Read the model definition and answer for the solid it produces. Units are mm, in the model's axes. Coordinates: 2 decimals unless noted, no trailing zeros. Order: outer loops, then holes, each group sorted by start corner. A loop starts at its lowest first (then second) coordinate and runs counter-clockwise, first axis right, second up. Notation, with made-up numbers: M 7,60.5 L 20,60.5 A13 cw 20,66.5 Z; hole C 2.5,-37 d5. An arc over 180 degrees is marked long. One line per question, with ' | ' between items. Start each with the question number.
1) Find section B-B, the plane z = -65. Write down the section's boundary in (x, y).
2) Find section A-A, the plane z = 0. Write down the section's boundary in (x, y).
3) Find section C-C, the plane z = -35.5. Write down the section's boundary in (x, y), plus the area to 3 significant figures.
4) Consider probe 1 along Z at (x, y) = (84.5, 0.3) (3 decimals); probe 2 along X at (y, z) = (0.75, 0); probe 3 along Z at (x, y) = (70.5, 0.45) (3 decimals). Determine where each line is inside the solid, lowest interval first.
from build123d import *

# Parameters (mm, degrees)
SKETCH6_R          = 1.6
EXTRUDE1_DEPTH     = 0.9
FILLET1_R          = 2
SKETCH9_R          = 0.925
CUT_EXTRUDE1_DEPTH = 1.9
CUT_EXTRUDE2_DEPTH = 1.9


with BuildPart() as part:
    # Sketch6 → Extrude1 (new body)
    with BuildSketch(Plane(origin=(0, 0, 0), x_dir=(1, 0, 0), z_dir=(0, 1, 0))):
        Polygon((-4.8675, 77.0686), (-4.8675, 62.335), (1.8535, 62.335), (1.8535, 12.335), (-4.8675, 12.335), (-4.8675, -10.395), (31.1875, -10.395), (31.1875, -7.244), (54.5375, -7.244), (54.5375, -10.395), (90.5925, -10.395), (90.5925, 25.66), (87.4415, 25.66), (87.4415, 49.01), (90.5925, 49.01), (90.5925, 83.6934), (78.5925, 83.6934), (78.5925, 80.9186), (19.1449, 80.9186), (19.1449, 75.196571572), (9.1325, 75.196571572), (5.1325, 77.0686), align=None)
        with Locations((0, 73.66)):
            Circle(SKETCH6_R, mode=Mode.SUBTRACT)
        with Locations((85.725, 76.2)):
            Circle(SKETCH6_R, mode=Mode.SUBTRACT)
        Circle(SKETCH6_R, mode=Mode.SUBTRACT)
        with Locations((85.725, -3.81)):
            Circle(SKETCH6_R, mode=Mode.SUBTRACT)
    extrude(amount=EXTRUDE1_DEPTH)

    # Fillet1
    fillet1_edges = [part.edges().sort_by_distance(p)[0] for p in [
        (5.1325, 0.45, -77.0686),
        (9.1325, 0.45, -75.196571572),
        (19.1449, 0.45, -75.196571572),
        (78.5925, 0.45, -80.9186),
        (90.5925, 0.45, -83.6934),
        (87.4415, 0.45, -49.01),
        (87.4415, 0.45, -25.66),
        (90.5925, 0.45, 10.395),
        (54.5375, 0.45, 7.244),
        (31.1875, 0.45, 7.244),
        (-4.8675, 0.45, 10.395),
        (1.8535, 0.45, -12.335),
        (1.8535, 0.45, -62.335),
        (-4.8675, 0.45, -77.0686),
    ]]
    fillet(fillet1_edges, radius=FILLET1_R)

    # Sketch9 → Cut-Extrude1 (cut, through all)
    with BuildSketch(Plane.XZ):
        with Locations((4.454560153, -47.705692794)):
            Circle(SKETCH9_R)
        with Locations((15.248482102, -49.222679594)):
            Circle(SKETCH9_R)
        with Locations((9.269949446, -13.442417616)):
            Circle(SKETCH9_R)
        with Locations((20.063871395, -14.959404416)):
            Circle(SKETCH9_R)
        with Locations((29.718985107, -16.316341854)):
            Circle(SKETCH9_R)
        with Locations((24.903595814, -50.579617033)):
            Circle(SKETCH9_R)
        with Locations((35.697517763, -52.096603833)):
            Circle(SKETCH9_R)
        with Locations((40.512907056, -17.833328655)):
            Circle(SKETCH9_R)
        with Locations((50.168020768, -19.190266093)):
            Circle(SKETCH9_R)
        with Locations((45.352631475, -53.453541271)):
            Circle(SKETCH9_R)
        with Locations((56.146553424, -54.970528072)):
            Circle(SKETCH9_R)
        with Locations((60.961942717, -20.707252893)):
            Circle(SKETCH9_R)
        with Locations((65.801667136, -56.32746551)):
            Circle(SKETCH9_R)
        with Locations((70.617056429, -22.064190332)):
            Circle(SKETCH9_R)
        with Locations((81.410978378, -23.581177132)):
            Circle(SKETCH9_R)
        with Locations((76.595589085, -57.844452311)):
            Circle(SKETCH9_R)
    extrude(amount=-CUT_EXTRUDE1_DEPTH, mode=Mode.SUBTRACT)

    # Sketch11 → Cut-Extrude2 (cut, through all)
    with BuildSketch(Plane(origin=(0, 0.9, 0), x_dir=(1, 0, 0), z_dir=(0, 1, 0))):
        with BuildLine():
            Line((88.342130657, 63.4125), (90.5925, 63.4125))
            Line((90.5925, 63.4125), (90.5925, 66.5875))
            Line((90.5925, 66.5875), (88.342130657, 66.5875))
            ThreePointArc((88.342130657, 66.5875), (82.4175, 65), (88.342130657, 63.4125))
        make_face()
    extrude(amount=-CUT_EXTRUDE2_DEPTH, mode=Mode.SUBTRACT)


solid = part.part
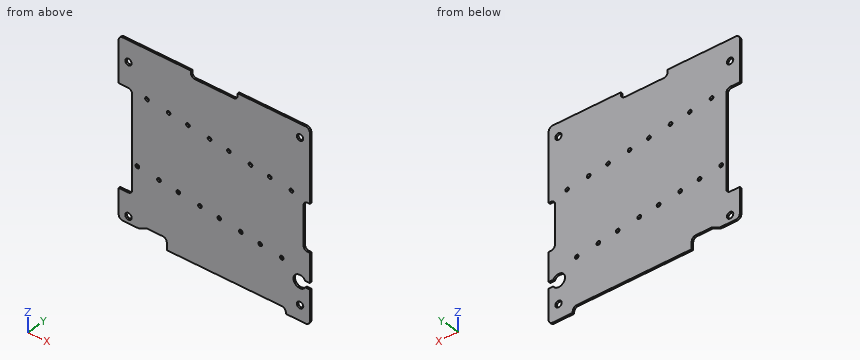
Report:
1) outline: M -4.87,0 L 82.42,0 L 82.42,0.9 L -4.87,0.9 Z
2) outline: M -4.87,0 L -1.6,0 L -1.6,0.9 L -4.87,0.9 Z; M 1.6,0 L 90.59,0 L 90.59,0.9 L 1.6,0.9 Z
3) outline: M 1.85,0 L 87.44,0 L 87.44,0.9 L 1.85,0.9 Z | area: 77.0 mm^2
4) probe 1: z = -83.693 to -77.229, -75.171 to -67.981, -62.019 to 2.781, 4.839 to 10.395 | probe 2: x = -4.87 to -1.6, 1.6 to 90.59 | probe 3: z = -80.919 to -22.982, -21.147 to 10.395
